```python
from build123d import *

# Parameters (mm, degrees)
SKETCH1_R           = 2.5
BOSS_EXTRUDE1_DEPTH = 3
BOSS_EXTRUDE2_DEPTH = 3


with BuildPart() as part:
    # Sketch1 → Boss-Extrude1 (new body)
    with BuildSketch(Plane(origin=(0, 0, 0), x_dir=(1, 0, 0), z_dir=(0, 1, 0))):
        with BuildLine():
            Line((-21, 66), (-16.439282223, 66))
            ThreePointArc((-16.439282223, 66), (-10.707167181, 67.805925486), (-7.045406667, 72.571428571))
            ThreePointArc((-7.045406667, 72.571428571), (0, 77.5), (7.045406667, 72.571428571))
            ThreePointArc((7.045406667, 72.571428571), (10.707167181, 67.805925486), (16.439282223, 66))
            Line((16.439282223, 66), (21, 66))
            ThreePointArc((21, 66), (24.535533906, 64.535533906), (26, 61))
            Line((26, 61), (26, 5))
            ThreePointArc((26, 5), (24.535533906, 1.464466094), (21, 0))
            Line((21, 0), (-21, 0))
            ThreePointArc((-21, 0), (-24.535533906, 1.464466094), (-26, 5))
            Line((-26, 5), (-26, 61))
            ThreePointArc((-26, 61), (-24.535533906, 64.535533906), (-21, 66))
        make_face()
        with Locations(Location((0, 70, 0), (0, 0, 270))):
            Circle(SKETCH1_R, mode=Mode.SUBTRACT)
    extrude(amount=BOSS_EXTRUDE1_DEPTH)

    # Sketch2 → Boss-Extrude2 (add)
    with BuildSketch(Plane.XZ):
        with BuildLine():
            Line((-10, -9), (10, -9))
            ThreePointArc((10, -9), (11.414213562, -8.414213562), (12, -7))
            Line((12, -7), (12, 1))
            ThreePointArc((12, 1), (11.414213562, 2.414213562), (10, 3))
            Line((10, 3), (-10, 3))
            ThreePointArc((-10, 3), (-11.414213562, 2.414213562), (-12, 1))
            Line((-12, 1), (-12, -7))
            ThreePointArc((-12, -7), (-11.414213562, -8.414213562), (-10, -9))
        make_face()
    extrude(amount=BOSS_EXTRUDE2_DEPTH)


solid = part.part
```
Input: part model. Units: mm. Frame: model coordinates. A direction names the side the tool comes from. Coordinates: 2 decimals unless noted, no trailing zeros. Loops run counter-clockwise (first coordinate to the right, second up) from the corner with the lowest first, then second, coordinate; pieces in that order, holes last. Notation, with made-up numbers: M -18,-20.5 L 0,-20.5 A17 cw 0,5.5 Z; hole C -1,-35.5 d11. An arc over 180 degrees is marked long. Use a Markdown table: item, result. Add a question column.
1) Line query: L1, parallel to Z at x = -20, y = 0.8; L2, parallel to Y at x = 15.5, z = -51; L3, parallel to X at y = 1.4, z = -70. Output: solid intervals per line, ascending. Write a range as from..to.
2) Pin query (flat end, axial travel): P1, Ø0.9, axis at x = -6, y = 1.5, coming from the +Z side; P2, Ø0.9, axis at y = -1.5, z = -2, coming from the -X side; P3, Ø2, axis at y = -2, z = -52.5, coming from the -X side; P4, Ø5, axis at x = 13, z = -35.5, coming from the -Y side. Return the tip coordinate at first contact, or that it passes through.
3) Section D-D, the plane z = -30. Return the cut outline in (x, y), plus the area to 3 significant figures.
4) Section A-A, the plane x = 0. Return the cut outline in (y, z).
5) Section B-B, the plane y = 1.3. Return the cut outline in (x, z), plus the area to 3 significant figures.
6) Draft query along X for faces 1 (the cylindrical face through (-1.5, 1.5, -72)), 2 (the cylindrical face through (25, 1, -2)), 3 (the flat face through (0, 1, 0)). Return one class per face: +X half, -X half, draft (parallel to the pull), parting line (faces both ways), or undercut.
7) Section C-C, the plane z = -70. Return the cut outline in (x, y), plus the area to 3 significant figures.
8) Set-up query: faces 4 (the flat face through (0, -1, -9)), 5 (the flat face through (-19, 1, -66)), 6 (the cylindrical face through (11.4, -1.48, -8.43)), 7 (the cylindrical face through (-11.43, -1.48, -8.4)), 8 (the flat face through (12, -1, -3)). Return all of +Z, -Z, +X, -X, +Y, -Y with unobstructed straight access to the full face (end or side cutting, diameter ignored); none if empty.
Answer below:
| question | item | result |
|---|---|---|
| 1 | L1 | -66..0 |
| 1 | L2 | 0..3 |
| 1 | L3 | -8.44..-2.5, 2.5..8.44 |
| 2 | P1 | z = 0 |
| 2 | P2 | x = -12 |
| 2 | P3 | through |
| 2 | P4 | y = 0 |
| 3 | outline | M -26,0 L 26,0 L 26,3 L -26,3 Z |
| 3 | area | 156 mm2 |
| 4 | outline | M -3,-9 L 0,-9 L 0,-67.5 L 3,-67.5 L 3,0 L 0,0 L 0,3 L -3,3 Z; M 0,-77.5 L 3,-77.5 L 3,-72.5 L 0,-72.5 Z |
| 5 | outline | M -26,-61 A5 ccw -21,-66 L -16.44,-66 A10 cw -7.05,-72.57 A7.5 ccw 7.05,-72.57 A10 cw 16.44,-66 L 21,-66 A5 ccw 26,-61 L 26,-5 A5 ccw 21,0 L -21,0 A5 ccw -26,-5 Z; hole C 0,-70 d5 |
| 5 | area | 3,570 mm2 |
| 6 | face 1 | undercut |
| 6 | face 2 | +X half |
| 6 | face 3 | draft |
| 7 | outline | M -8.44,0 L -2.5,0 L -2.5,3 L -8.44,3 Z; M 2.5,0 L 8.44,0 L 8.44,3 L 2.5,3 Z |
| 7 | area | 35.6 mm2 |
| 8 | face 4 | -Z, +X, -X, -Y |
| 8 | face 5 | -Z, -X, +Y, -Y |
| 8 | face 6 | -Z, +X, -Y |
| 8 | face 7 | -Z, -X, -Y |
| 8 | face 8 | +Z, -Z, +X, -Y |
